```python
from build123d import *

# Parameters (mm, degrees)
EXTRUDE_1_DEPTH     = 10.3
SKETCH_2_R          = 1.4
EXTRUDE_2_DEPTH     = 5.8
CHAMFER_1_SIZE      = 0.5
SKETCH_3_R          = 1.4
CUT_EXTRUDE_1_DEPTH = 7


with BuildPart() as part:
    # Эскиз1 → Бобышка-Вытянуть1 (new body)
    with BuildSketch(Plane(origin=(0, 0, 0), x_dir=(1, 0, 0), z_dir=(0, 1, 0))):
        Polygon((0, 2.886751346), (-2.5, 1.443375673), (-2.5, -1.443375673), (0, -2.886751346), (2.5, -1.443375673), (2.5, 1.443375673), align=None)
    extrude(amount=EXTRUDE_1_DEPTH)

    # Эскиз2 → Бобышка-Вытянуть2 (add)
    with BuildSketch(Plane.XZ):
        with Locations(Location((0, 0, 0), (0, 0, 270))):
            Circle(SKETCH_2_R)
    extrude(amount=EXTRUDE_2_DEPTH)

    # Фаска1
    chamfer_1_edges = [part.edges().sort_by_distance(p)[0] for p in [
        (0, -5.8, 1.4),
    ]]
    chamfer(chamfer_1_edges, length=CHAMFER_1_SIZE)

    # Эскиз3 → Вырез-Вытянуть1 (cut)
    with BuildSketch(Plane(origin=(0, 10.3, 0), x_dir=(1, 0, 0), z_dir=(0, 1, 0))):
        with Locations(Location((0, 0, 0), (0, 0, 90))):
            Circle(SKETCH_3_R)
    extrude(amount=-CUT_EXTRUDE_1_DEPTH, mode=Mode.SUBTRACT)


solid = part.part
```
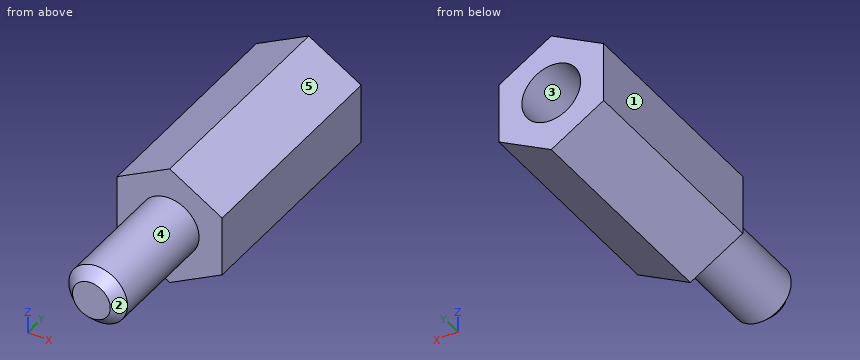
Geometry: final body of the model. Coordinates: model frame, mm. Face numbers are marked on the shaded views. A direction names the side the tool comes from. Round coordinates to 2 decimals unless told otherwise and drop trailing zeros. Order: outer loops, then holes, each group sorted by start corner. A loop starts at its lowest first (then second) coordinate and runs counter-clockwise, first axis right, second up. Notation, with made-up numbers: (65, 4.5) - (112, 4.5) arc R32 cw to (112, 43.5) - close; hole circle Ø11 at (-11.5, -29). An arc over 180 degrees is marked (long way). Use CSV: the item, a comma, the result in double quotes. Start each with the question number.
Q1. Section query A-A (y = 4.5). Return loops of the section in (x, z), and give its area (3 significant figures).
Q2. Mould query, pull axis Z, two halves, no side actions, for the marked faces 1, 2 and 3. Classes: +Z half, -Z half, draft (parallel to the pull), parting line (faces both ways), or undercut.
Q3. Material intervals for line 1 along X through (y, z) = (7.25, 0); line 2 along X through (y, z) = (-3.5, -0.05); line 3 along Y through (x, z) = (-1.4, -0.5), sorted ascending. Write a range as from..to.
Q4. Section query B-B (z = 0). Return loops of the section in (x, y), and give its area (3 significant figures).
Q5. Access query for the marked faces 4 and 5. Directions: +Z, -Z, +X, -X, +Y, -Y. A direction counts if a zero-diameter tool reaches every point of the face in a straight line with its end or side. Return the directions, or none.
Q6. First-contact query: pin 1 (1.4 mm diameter, centred on x = 0.5, z = 0, fed in from +Y); pin 2 (1.5 mm diameter, centred on y = -4, z = 1, fed in from +X). Flat tips, straight axial feed; report the tip coordinate or a pass-through.
Q7. Section query D-D (z = 2.4). Return loops of the section in (x, y), and give its area (3 significant figures).
Q8. Section query C-C (y = -1.75). Return loops of the section in (x, z), and give its area (3 significant figures).
Result set:
1,outline,"(-2.5, -1.44) - (0, -2.89) - (2.5, -1.44) - (2.5, 1.44) - (0, 2.89) - (-2.5, 1.44) - close; hole circle Ø2.8 at (0, 0)"
1,area,"15.5 mm2"
2,face 1,"draft"
2,face 2,"parting line"
2,face 3,"undercut"
3,line 1,"x = -2.5..-1.4, 1.4..2.5"
3,line 2,"x = -1.4..1.4"
3,line 3,"y = 0..10.3"
4,outline,"(-2.5, 0) - (-1.4, 0) - (-1.4, -5.3) - (-0.9, -5.8) - (0.9, -5.8) - (1.4, -5.3) - (1.4, 0) - (2.5, 0) - (2.5, 10.3) - (1.4, 10.3) - (1.4, 3.3) - (-1.4, 3.3) - (-1.4, 10.3) - (-2.5, 10.3) - close"
4,area,"47.9 mm2"
5,face 4,"-Y"
5,face 5,"+Z, +X, +Y, -Y"
6,pin 1,"stops at y = 3.3"
6,pin 2,"stops at x = 1.38"
7,outline,"(-0.84, 0) - (0.84, 0) - (0.84, 10.3) - (-0.84, 10.3) - close"
7,area,"17.4 mm2"
8,outline,"circle Ø2.8 at (0, 0)"
8,area,"6.16 mm2"
